from build123d import *

# Parameters (mm, degrees)
F0_W           = 31.75
F0_H           = 38.1
F1_DEPTH       = 19.05
F3_DEPTH       = 19.051
F5_DEPTH       = 18.9707249215
F7_DEPTH       = 18.9707249215
F9_DEPTH       = 25.4
F12_DEPTH      = 14.5164068706
F12_DEPTH_BACK = 14.5164068706


with BuildPart() as f1:
    # F0 (on Right) → F1 (new body)
    with BuildSketch(Plane.YZ):
        Rectangle(F0_W, F0_H)
    extrude(amount=F1_DEPTH)

    # F2 (on face) → F3 (cut, through all)
    with BuildSketch(Plane.YZ.offset(19.05)):
        Polygon((15.875, 19.05), (0, 19.05), (15.875, 9.2454001677), align=None)
        Polygon((-15.875, 9.2454001677), (0, 19.05), (-15.875, 19.05), align=None)
        Polygon((-15.875, -19.05), (15.875, -19.05), (15.875, 6.5585523178), (0, 16.3631521501), (-15.875, 6.5585523178), align=None)
    extrude(amount=-F3_DEPTH, mode=Mode.SUBTRACT)

    # F4 (on face) → F5 (cut, through all)
    with BuildSketch(Plane(origin=(0, -8.5168191059, 13.7899053117), x_dir=(1, 0, 0), z_dir=(0, -0.5254716511, 0.8508111094))):
        Polygon((19.05, -10.060293047), (19.05, 16.251566953), (-0.0666852809, -10.060293047), align=None)
    extrude(amount=-F5_DEPTH, mode=Mode.SUBTRACT)

    # F6 (on face) → F7 (cut, through all)
    with BuildSketch(Plane(origin=(0, 8.5168191059, 13.7899053117), x_dir=(1, 0, 0), z_dir=(0, 0.5254716511, 0.8508111094))):
        Polygon((125.3145152414, -10.0102349529), (125.3145152414, 10.060293047), (110.7324230899, 10.060293047), align=None)
    extrude(amount=-F7_DEPTH, mode=Mode.SUBTRACT)

    # F8 (on face) → F9 (cut)
    with BuildSketch(Plane(origin=(0, 8.5168191059, 13.7899053117), x_dir=(1, 0, 0), z_dir=(0, 0.5254716511, 0.8508111094))):
        Polygon((-0.0666852809, 10.060293047), (19.05, -16.251566953), (19.05, 10.060293047), align=None)
    extrude(amount=-F9_DEPTH, mode=Mode.SUBTRACT)

    # F10: F1 across plane


with BuildPart() as f1_1:
    add(f1.part)
    add(f1.part.mirror(Plane.YZ))

    # F11 (on Right) → F12 (cut, two sides)
    with BuildSketch(Plane.YZ) as f12_sk:
        Polygon((-15.875, 9.2454001677), (-15.875, 6.5585523178), (-3.175, 14.4022321837), (-3.175, 17.0890800335), align=None)
        Polygon((15.875, 9.2454001677), (3.175, 17.0890800335), (3.175, 14.4022321837), (15.875, 6.5585523178), align=None)
    extrude(amount=-F12_DEPTH, mode=Mode.SUBTRACT)
    extrude(f12_sk.sketch, amount=F12_DEPTH_BACK, mode=Mode.SUBTRACT)


solid = f1_1.part
The model under review builds one solid part; all positions refer to its coordinate system, in mm. A direction names the side the tool comes from. Coordinates: 2 decimals unless noted, no trailing zeros. Write each loop counter-clockwise with the first axis right and the second up, starting at its lowest first coordinate (ties: lowest second). Pieces come first, ordered by that corner, then holes. Notation, with made-up numbers: (44, 72.5) -> (97, 72.5) arc R18 cw to (97, 103.5) -> close; hole circle Ø8 at (64.5, 39). An arc over 180 degrees is marked (long way). Answer in a Markdown table with one row per item.
1. We need section D-D, the plane y = -2. State the section outline as (x, z) points.
Answers below:
| item | result |
|---|---|
| outline | (-12.81, 17.81) -> (-11.78, 15.13) -> (11.78, 15.13) -> (12.81, 17.81) -> close |
2. We need section A-A, the plane z = 16. State the section outline as (x, y) points (3 decimals), and give its area (3 significant figures).
Answers below:
| item | result |
|---|---|
| outline | (-12.988, -0.588) -> (-11.388, -3.175) -> (11.388, -3.175) -> (12.988, -0.588) -> close; (-12.988, 0.588) -> (12.988, 0.588) -> (11.388, 3.175) -> (-11.388, 3.175) -> close |
| area | 126 mm^2 |
3. Wall thickness on probe 1 along Y at (x, z) = (1, 16.25) (3 decimals); probe 2 along Y at (x, z) = (-1.75, 15.35) (3 decimals); probe 3 along Z at (x, y) = (10.25, -2.75): over which ranges is each line inside the solid? List them lowest first. Write a range as [from, to].
Answers below:
| item | result |
|---|---|
| probe 1 | y = [-3.175, -0.183], [0.183, 3.175] |
| probe 2 | y = [-3.175, -1.64], [1.64, 3.175] |
| probe 3 | z = [14.66, 17.35] |
4. We need section B-B, the plane x = -8.75. State the section outline as (y, z) points (3 decimals).
Answers below:
| item | result |
|---|---|
| outline | (-3.175, 14.402) -> (0, 16.363) -> (3.175, 14.402) -> (3.175, 17.089) -> (0, 19.05) -> (-3.175, 17.089) -> close |
5. For faces 1 (the flat face through (-0.203, -1.61, 18.056)), 2 (the flat face through (-0.189, -1.565, 15.396)), list the 3-axis set-ups (+Z, -Z, +X, -X, +Y, -Y) from which the entire face can be reached by the end or side of a thin tool; tool diameter is ignored.
Answers below:
| item | result |
|---|---|
| face 1 | +Z, +X, -X, -Y |
| face 2 | -Z, +X, -X |
6. We need section C-C, the plane z = 14.75. State the section outline as (x, y) points (3 decimals).
Answers below:
| item | result |
|---|---|
| outline | (-11.259, -2.612) -> (-10.911, -3.175) -> (10.911, -3.175) -> (11.259, -2.612) -> close; (-11.259, 2.612) -> (11.259, 2.612) -> (10.911, 3.175) -> (-10.911, 3.175) -> close |
7. Clearance check with flat-ended pins moving along their axes: pin 1 Ø1.5 at (x, y) = (6.5, 1.5) entering from +Z; pin 2 Ø1.5 at (x, z) = (-3.5, 18) entering from +Y. State where each tip first meets the part, or that it passes through.
Answers below:
| item | result |
|---|---|
| pin 1 | stops at z = 18.59 |
| pin 2 | stops at y = 2.91 |
